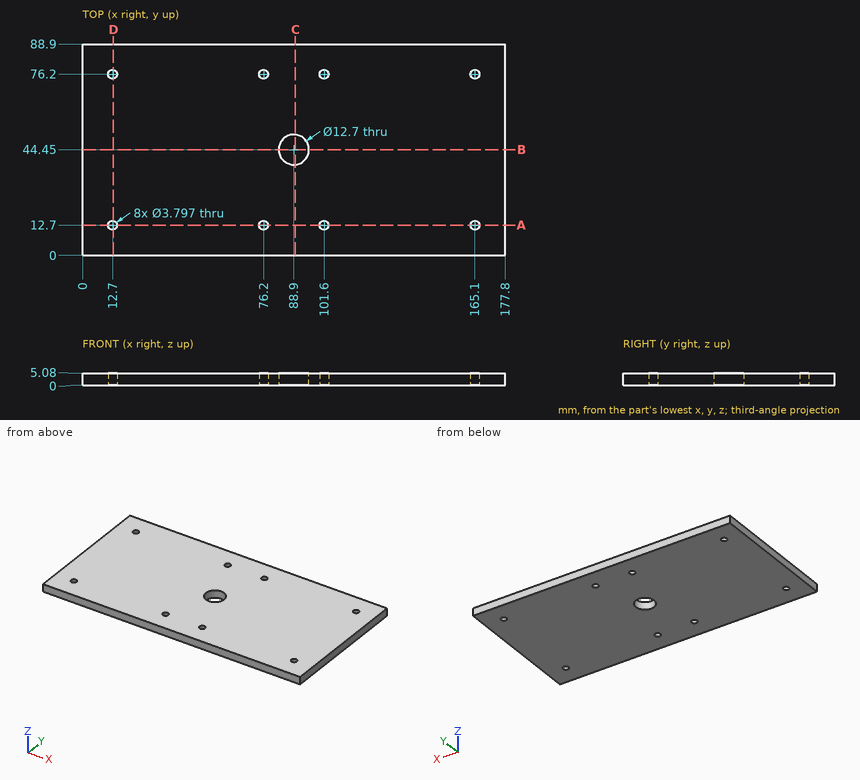
Design review of the part shown in the three views and the two pictorial views. Dimensions are in mm from the part's minimum x, y and z. Give positions to 0.01 mm unless a question says otherwise; leave off trailing zeros. Write each loop counter-clockwise with the first axis right and the second up, starting at its lowest first coordinate (ties: lowest second). Pieces come first, ordered by that corner, then holes. Notation, with made-up numbers: (28.25, -24) - (33.25, -24) arc R18 ccw to (33.25, 9) - close; hole circle Ø6 at (10.25, 29.25). An arc over 180 degrees is marked (long way). Return JSON: item names as keys, results as strings. Group by question number.
(1) We need section B-B, the plane y = 44.45. Give the boundary of the cut face in (x, z).
(2) We need section D-D, the plane x = 13. Give the boundary of the cut face in (y, z) (1 decimal).
(3) We need section C-C, the plane x = 89.5. Give the boundary of the cut face in (y, z), then the cut area to 3 significant figures.
(4) To check wall thickness, follow probe 1 along X at (y, z) = (76.2, 3.4); probe 2 along Y at (x, z) = (12.7, 2.3); probe 3 along X at (y, z) = (11, 2.5) (1 decimal). State the ranges of each line that lie inside material, in increasing order.
(5) We need section A-A, the plane y = 12.7. Give the boundary of the cut face in (x, z), then the cut area to 3 significant figures.
(6) Insertion check: pin 1 (5 mm diameter, centred on x = 165.1, y = 12.7, fed in from -Z). The pin has a flat end and moves straight along its axis. Give the tip position at first contact, or say it passes through.
Reported:
{
 "1": {"outline": "(0, 0) - (82.55, 0) - (82.55, 5.08) - (0, 5.08) - close; (95.25, 0) - (177.8, 0) - (177.8, 5.08) - (95.25, 5.08) - close"},
 "2": {"outline": "(0, 0) - (10.8, 0) - (10.8, 5.1) - (0, 5.1) - close; (14.6, 0) - (74.3, 0) - (74.3, 5.1) - (14.6, 5.1) - close; (78.1, 0) - (88.9, 0) - (88.9, 5.1) - (78.1, 5.1) - close"},
 "3": {"outline": "(0, 0) - (38.13, 0) - (38.13, 5.08) - (0, 5.08) - close; (50.77, 0) - (88.9, 0) - (88.9, 5.08) - (50.77, 5.08) - close", "area": "387 mm2"},
 "4": {"probe 1": "x = 0 to 10.8, 14.6 to 74.3, 78.1 to 99.7, 103.5 to 163.2, 167 to 177.8", "probe 2": "y = 0 to 10.8, 14.6 to 74.3, 78.1 to 88.9", "probe 3": "x = 0 to 11.9, 13.5 to 75.4, 77 to 100.8, 102.4 to 164.3, 165.9 to 177.8"},
 "5": {"outline": "(0, 0) - (10.8, 0) - (10.8, 5.08) - (0, 5.08) - close; (14.6, 0) - (74.3, 0) - (74.3, 5.08) - (14.6, 5.08) - close; (78.1, 0) - (99.7, 0) - (99.7, 5.08) - (78.1, 5.08) - close; (103.5, 0) - (163.2, 0) - (163.2, 5.08) - (103.5, 5.08) - close; (167, 0) - (177.8, 0) - (177.8, 5.08) - (167, 5.08) - close", "area": "826 mm2"},
 "6": {"pin 1": "stops at z = 0"}
}
